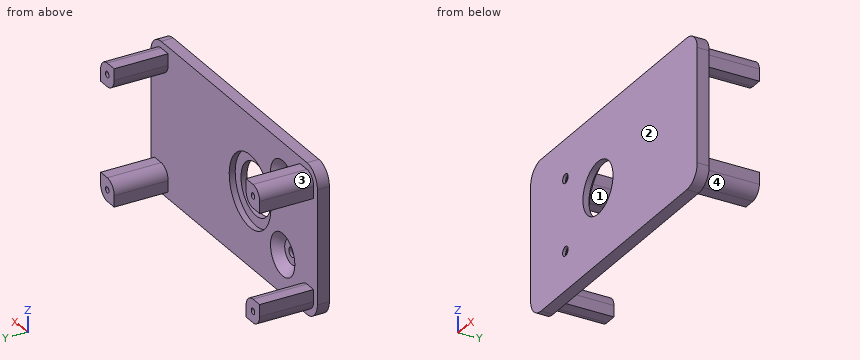
from build123d import *

# Parameters (mm, degrees)
SKETCH1_W           = 121.92
SKETCH1_H           = 63.5
BOSS_EXTRUDE1_DEPTH = 5.08
FILLET1_R           = 7.62
SKETCH2_W           = 9.906
SKETCH2_H           = 9.906
BOSS_EXTRUDE2_DEPTH = 22.86
FILLET2_R           = 4.826
FILLET3_R           = 5.08
SKETCH3_R           = 1.27
CUT_EXTRUDE1_DEPTH  = 22.86
CUT_EXTRUDE2_REACH  = 142.276
SKETCH5_R           = 10.9982
CUT_EXTRUDE3_REACH  = 142.276
SKETCH6_R           = 1.9939
SKETCH7_R           = 5.08
CUT_EXTRUDE4_DEPTH  = 3.81
CHAMFER1_SIZE       = 3.81
SKETCH8_R           = 15.24
CUT_EXTRUDE5_DEPTH  = 2.54


with BuildPart() as part:
    # Sketch1 → Boss-Extrude1 (new body)
    with BuildSketch(Plane(origin=(0, 0, 0), x_dir=(1, 0, 0), z_dir=(0, 1, 0))):
        with Locations((60.96, 31.75)):
            Rectangle(SKETCH1_W, SKETCH1_H)
    extrude(amount=BOSS_EXTRUDE1_DEPTH)

    # Fillet1
    fillet1_edges = [part.edges().sort_by_distance(p)[0] for p in [
        (0, 2.54, -63.5),
        (121.92, 2.54, -63.5),
        (121.92, 2.54, 0),
        (0, 2.54, 0),
    ]]
    fillet(fillet1_edges, radius=FILLET1_R)

    # Sketch2 → Boss-Extrude2 (add)
    with BuildSketch(Plane(origin=(0, 5.08, 0), x_dir=(1, 0, 0), z_dir=(0, 1, 0))):
        with Locations((7.747, 55.753)):
            Rectangle(SKETCH2_W, SKETCH2_H)
        with Locations((114.173, 55.753)):
            Rectangle(SKETCH2_W, SKETCH2_H)
        with Locations((114.173, 7.747)):
            Rectangle(SKETCH2_W, SKETCH2_H)
        with Locations((7.747, 7.747)):
            Rectangle(SKETCH2_W, SKETCH2_H)
    extrude(amount=BOSS_EXTRUDE2_DEPTH)

    # Fillet2
    fillet2_edges = [part.edges().sort_by_distance(p)[0] for p in [
        (2.794, 16.51, -60.706),
        (119.126, 16.51, -60.706),
        (119.126, 16.51, -2.794),
        (2.794, 16.51, -2.794),
    ]]
    fillet(fillet2_edges, radius=FILLET2_R)

    # Fillet3
    fillet3_edges = [part.edges().sort_by_distance(p)[0] for p in [
        (12.7, 16.51, -50.8),
        (109.22, 16.51, -50.8),
        (109.22, 16.51, -12.7),
        (12.7, 16.51, -12.7),
    ]]
    fillet(fillet3_edges, radius=FILLET3_R)

    # Sketch3 → Cut-Extrude1 (cut)
    with BuildSketch(Plane(origin=(0, 27.94, 0), x_dir=(1, 0, 0), z_dir=(0, 1, 0))):
        with Locations(Location((7.62, 55.88, 0), (0, 0, 270))):
            Circle(SKETCH3_R)
        with Locations(Location((114.3, 55.88, 0), (0, 0, 270))):
            Circle(SKETCH3_R)
        with Locations(Location((114.3, 7.62, 0), (0, 0, 270))):
            Circle(SKETCH3_R)
        with Locations(Location((7.62, 7.62, 0), (0, 0, 270))):
            Circle(SKETCH3_R)
    extrude(amount=-CUT_EXTRUDE1_DEPTH, mode=Mode.SUBTRACT)

    # Sketch5 → Cut-Extrude2 (cut, up to next)
    with BuildSketch(Plane.XZ, mode=Mode.PRIVATE) as cut_extrude2_sk1:
        with Locations(Location((49.276, -31.75, 0), (0, 0, 270))):
            Circle(SKETCH5_R)
    cut_extrude2_tool1 = extrude(cut_extrude2_sk1.sketch, amount=-CUT_EXTRUDE2_REACH, mode=Mode.PRIVATE) & part.part
    add(cut_extrude2_tool1.solids().sort_by_distance((49.276, 0, -31.75))[0], mode=Mode.SUBTRACT)

    # Sketch6 → Cut-Extrude3 (cut, up to next)
    with BuildSketch(Plane.XZ, mode=Mode.PRIVATE) as cut_extrude3_sk1:
        with Locations(Location((25.4, -16.51, 0), (0, 0, 270))):
            Circle(SKETCH6_R)
    cut_extrude3_tool1 = extrude(cut_extrude3_sk1.sketch, amount=-CUT_EXTRUDE3_REACH, mode=Mode.PRIVATE) & part.part
    # Sketch6 → Cut-Extrude3 (cut, up to next)
    with BuildSketch(Plane.XZ, mode=Mode.PRIVATE) as cut_extrude3_sk2:
        with Locations(Location((25.4, -46.99, 0), (0, 0, 270))):
            Circle(SKETCH6_R)
    cut_extrude3_tool2 = extrude(cut_extrude3_sk2.sketch, amount=-CUT_EXTRUDE3_REACH, mode=Mode.PRIVATE) & part.part
    add(cut_extrude3_tool1.solids().sort_by_distance((25.4, 0, -16.51))[0], mode=Mode.SUBTRACT)
    add(cut_extrude3_tool2.solids().sort_by_distance((25.4, 0, -46.99))[0], mode=Mode.SUBTRACT)

    # Sketch7 → Cut-Extrude4 (cut)
    with BuildSketch(Plane(origin=(0, 5.08, 0), x_dir=(1, 0, 0), z_dir=(0, 1, 0))):
        with Locations(Location((25.4, 46.99, 0), (0, 0, 270))):
            Circle(SKETCH7_R)
        with Locations(Location((25.4, 16.51, 0), (0, 0, 270))):
            Circle(SKETCH7_R)
    extrude(amount=-CUT_EXTRUDE4_DEPTH, mode=Mode.SUBTRACT)

    # Chamfer1
    chamfer1_edges = [part.edges().sort_by_distance(p)[0] for p in [
        (25.4, 5.08, -52.07),
        (25.4, 5.08, -21.59),
    ]]
    chamfer(chamfer1_edges, length=CHAMFER1_SIZE - 0.0001)  # a hair under: the kernel refuses the full size

    # Sketch8 → Cut-Extrude5 (cut)
    with BuildSketch(Plane(origin=(0, 5.08, 0), x_dir=(1, 0, 0), z_dir=(0, 1, 0))):
        with Locations(Location((49.276, 31.75, 0), (0, 0, 270))):
            Circle(SKETCH8_R)
    extrude(amount=-CUT_EXTRUDE5_DEPTH, mode=Mode.SUBTRACT)


solid = part.part
Geometry check sheet. Reference: the model listing, model coordinates, mm. Face numbers are marked on the shaded views. Give positions to 0.01 mm unless a question says otherwise; leave off trailing zeros. Loops run counter-clockwise (first coordinate to the right, second up) from the corner with the lowest first, then second, coordinate; pieces in that order, holes last. Notation, with made-up numbers: M 9.25,81.25 L 65.25,81.25 A10 cw 65.25,89.25 Z; hole C 33.5,-14 d5. An arc over 180 degrees is marked long. Answer as a JSON object with one key per item and string values. Group by question number.
Item 1: Sectioned sample at D-D on x = 98. Record the boundary of the cut face in (y, z), plus the area to 3 significant figures.
Item 2: Sectioned sample at A-A on y = 6.5. Record the boundary of the cut face in (x, z).
Item 3: Sectioned sample at C-C on x = 25.4. Give the number of separate pieces and of enclosed holes in the cut face, plus the area to 3 significant figures.
Item 4: Mould release check, pull along X, two halves, no side actions. Record for the marked faces 1, 2, 3 and 4: pulls with the +X half, pulls with the -X half, needs draft (parallel to the pull), parting line crosses it, or undercut.
Item 5: Gauge pin test, flat ends, axial feed: pin 1 (1.5 mm diameter, centred on y = 11, z = -48.5, fed in from +X); pin 2 (9 mm diameter, centred on x = 25.4, z = -16.51, fed in from +Y); pin 3 (0.8 mm diameter, centred on x = 115, z = -8, fed in from +Y); pin 4 (4 mm diameter, centred on x = 5, y = 22, fed in from +Z). Record the tip position at first contact, or that the pin passes through.
Item 6: Sectioned sample at B-B on z = -31.75. Record the boundary of the cut face in (x, y), plus the area to 3 significant figures.
Item 7: Material ranges on L1, parallel to X at y = 0.7, z = -16.51; L2, parallel to X at y = 4.05, z = -31.75; L3, parallel to X at y = 25, z = -55.5, recorded low to high.
Findings below:
{
 "1": {"outline": "M 0,-63.5 L 5.08,-63.5 L 5.08,0 L 0,0 Z", "area": "323 mm2"},
 "2": {"outline": "M 2.79,-55.88 A4.83 ccw 7.62,-60.71 L 12.7,-60.71 L 12.7,-55.88 A5.08 ccw 7.62,-50.8 L 2.79,-50.8 Z; M 2.79,-12.7 L 7.62,-12.7 A5.08 ccw 12.7,-7.62 L 12.7,-2.79 L 7.62,-2.79 A4.83 ccw 2.79,-7.62 Z; M 109.22,-60.71 L 114.3,-60.71 A4.83 ccw 119.13,-55.88 L 119.13,-50.8 L 114.3,-50.8 A5.08 ccw 109.22,-55.88 Z; M 109.22,-7.62 A5.08 ccw 114.3,-12.7 L 119.13,-12.7 L 119.13,-7.62 A4.83 ccw 114.3,-2.79 L 109.22,-2.79 Z; hole C 7.62,-55.88 d2.54; hole C 7.62,-7.62 d2.54; hole C 114.3,-55.88 d2.54; hole C 114.3,-7.62 d2.54"},
 "3": {"separate pieces": "3", "enclosed holes": "0", "area": "206 mm2"},
 "4": {"face 1": "undercut", "face 2": "needs draft", "face 3": "pulls with the -X half", "face 4": "pulls with the +X half"},
 "5": {"pin 1": "through", "pin 2": "y = 1.27", "pin 3": "y = 5.08", "pin 4": "z = -2.83"},
 "6": {"outline": "M 0,0 L 38.28,0 L 38.28,2.54 L 34.04,2.54 L 34.04,5.08 L 0,5.08 Z; M 60.27,0 L 121.92,0 L 121.92,5.08 L 64.52,5.08 L 64.52,2.54 L 60.27,2.54 Z", "area": "486 mm2"},
 "7": {"L1": "0 to 23.41, 27.39 to 121.92", "L2": "0 to 34.04, 64.52 to 121.92", "L3": "2.79 to 6.41, 8.83 to 12.69, 109.23 to 113.09, 115.51 to 119.13"}
}
